Read the model definition and answer for the solid it produces. Units are mm, in the model's axes. A direction names the side the tool comes from. Round coordinates to 2 decimals unless told otherwise and drop trailing zeros. Loops run counter-clockwise (first coordinate to the right, second up) from the corner with the lowest first, then second, coordinate; pieces in that order, holes last. Notation, with made-up numbers: M 13.25,71.25 L 29.25,71.25 A30 ccw 29.25,97.25 Z; hole C 7,53 d8. An arc over 180 degrees is marked long. Write each question's results on one line, items separated by ' | '.
from build123d import *

# Parameters (mm, degrees)
F1_DEPTH = 50.8
F2_W     = 254
F2_H     = 50.8
F3_DEPTH = 127


with BuildPart() as f1:
    # F0 (on Top) → F1 (new body)
    with BuildSketch(Plane.XY):
        Polygon((-330.2, 0), (0, 0), (254, 0), (254, 508), (0, 508), (-330.2, 508), align=None)
    extrude(amount=F1_DEPTH)

    # F2 (on face) → F3 (join)
    with BuildSketch(Plane.YZ.offset(254)):
        with Locations((254, 25.4)):
            Rectangle(F2_W, F2_H)
    extrude(amount=F3_DEPTH)


solid = f1.part
Item 1: The part is cut by section B-B (x = 272). Determine the outline of the cut face in (y, z), plus the area to 3 significant figures.
Outcome:
outline: M 127,0 L 381,0 L 381,50.8 L 127,50.8 Z | area: 12,900 mm2
Item 2: The part is cut by section A-A (z = 19). Determine the outline of the cut face in (x, y).
Outcome:
outline: M -330.2,0 L 254,0 L 254,127 L 381,127 L 381,381 L 254,381 L 254,508 L -330.2,508 Z
Item 3: For faces 1 (the face through (254, 63, 25)), 2 (the face through (-330.2, 258, 25)), 3 (the face through (317, 381, 25)), determine the directions among +Z, -Z, +X, -X, +Y, -Y from which every point of the face is accessible in a straight line to the end or side of a thin tool.
Outcome:
face 1: +Z, -Z, +X, -Y | face 2: +Z, -Z, -X, +Y, -Y | face 3: +Z, -Z, +X, +Y
Item 4: Straight lines are drawn through the part: line 1 (X direction, y = 71.5, z = 47.5); line 2 (Y direction, x = 304, z = 21.5). For each, find the intervals that lie inside material, in ascending order.
Outcome:
line 1: x = -330.2 to 254 | line 2: y = 127 to 381
Item 5: The part is cut by section C-C (y = 415). Determine the outline of the cut face in (x, z), plus the area to 3 significant figures.
Outcome:
outline: M -330.2,0 L 254,0 L 254,50.8 L -330.2,50.8 Z | area: 29,700 mm2
Item 6: Flat-ended cylindrical pins translate along their axes: pin 1 (3 mm diameter, centred on x = 22, z = 39, fed in from -Y); pin 2 (15 mm diameter, centred on y = 416.5, z = 13, fed in from +X). Find the tip coordinate at first contact, or state that the pin passes through.
Outcome:
pin 1: stops at y = 0 | pin 2: stops at x = 254
